Check sheet for the modelled part. Datum: model origin and axes. Units: mm. Face numbers are marked on the shaded views. Give positions to 0.01 mm unless a question says otherwise; leave off trailing zeros. Order: outer loops, then holes, each group sorted by start corner. A loop starts at its lowest first (then second) coordinate and runs counter-clockwise, first axis right, second up.
from build123d import *

# Parameters (mm, degrees)
F3_DEPTH = 1.27


with BuildPart() as f1:
    # F0 (on Front) → F1 (revolve)
    with BuildSketch(Plane.XZ):
        with BuildLine():
            Line((-6.985, 6.35), (-6.985, 0))
            Line((-6.985, 0), (-3.81, 0))
            ThreePointArc((-3.81, 0), (-2.6940768363, 2.6940768363), (0, 3.81))
            Line((0, 3.81), (0, 6.35))
            Line((0, 6.35), (-6.985, 6.35))
        make_face()
    revolve(axis=Axis((0, 0, 5.08), (0, 0, 1)))

    # F2 (on face) → F3 (cut)
    with BuildSketch(Plane.XY.offset(6.35)):
        with BuildLine():
            Line((-5.0499272347, 4.825811841), (5.0499272347, 4.825811841))
            ThreePointArc((5.0499272347, 4.825811841), (0, 6.985), (-5.0499272347, 4.825811841))
        make_face()
        with BuildLine():
            Line((5.0499272347, -4.825811841), (5.0499272347, 4.825811841))
            Line((5.0499272347, 4.825811841), (-5.0499272347, 4.825811841))
            Line((-5.0499272347, 4.825811841), (-5.0499272347, -4.825811841))
            Line((-5.0499272347, -4.825811841), (-1.3193129815, -4.825811841))
            add(Edge.make_bspline(
                [(-1.3193129815, -4.825811841), (-2.5203953314, -4.5677027566), (-3.3083202269, -3.8047253512)],
                knots=[0.3382919108, 0.3382919108, 0.3382919108, 1, 1, 1], degree=2))
            add(Edge.make_bspline(
                [(-3.3083202269, -3.8047253512), (-4.4990641643, -2.6516830689), (-4.4990641643, -0.5382958521)],
                knots=[0, 0, 0, 1, 1, 1], degree=2))
            add(Edge.make_bspline(
                [(-4.4990641643, -0.5382958521), (-4.4990641643, 1.7656941762), (-3.3439273456, 2.9082637766)],
                knots=[0, 0, 0, 1, 1, 1], degree=2))
            add(Edge.make_bspline(
                [(-3.3439273456, 2.9082637766), (-2.1887905268, 4.0508333769), (0.0418907278, 4.0508333769)],
                knots=[0, 0, 0, 1, 1, 1], degree=2))
            add(Edge.make_bspline(
                [(0.0418907278, 4.0508333769), (1.6400219928, 4.0508333769), (3.1250482929, 3.6570605358)],
                knots=[0, 0, 0, 1, 1, 1], degree=2))
            Line((3.1250482929, 3.6570605358), (3.1250482929, 1.7719777854))
            Line((3.1250482929, 1.7719777854), (2.6872901875, 1.7719777854))
            Line((2.6872901875, 1.7719777854), (2.5092545944, 2.8590421714))
            add(Edge.make_bspline(
                [(2.5092545944, 2.8590421714), (2.0589292707, 3.179506239), (1.4274265493, 3.3533527593)],
                knots=[0, 0, 0, 1, 1, 1], degree=2))
            add(Edge.make_bspline(
                [(1.4274265493, 3.3533527593), (0.7959238279, 3.5271992796), (0.0942541375, 3.5271992796)],
                knots=[0, 0, 0, 1, 1, 1], degree=2))
            add(Edge.make_bspline(
                [(0.0942541375, 3.5271992796), (-1.5813749739, 3.5271992796), (-2.356353438, 2.5281054219)],
                knots=[0, 0, 0, 1, 1, 1], degree=2))
            add(Edge.make_bspline(
                [(-2.356353438, 2.5281054219), (-3.131331902, 1.5290115642), (-3.131331902, -0.5257286337)],
                knots=[0, 0, 0, 1, 1, 1], degree=2))
            add(Edge.make_bspline(
                [(-3.131331902, -0.5257286337), (-3.131331902, -2.4568911847), (-2.3333135377, -3.4549377742)],
                knots=[0, 0, 0, 1, 1, 1], degree=2))
            add(Edge.make_bspline(
                [(-2.3333135377, -3.4549377742), (-1.5352951734, -4.4529843637), (0.0293235095, -4.4529843637)],
                knots=[0, 0, 0, 1, 1, 1], degree=2))
            add(Edge.make_bspline(
                [(0.0293235095, -4.4529843637), (0.5801865798, -4.4529843637), (1.1823657918, -4.3220758394)],
                knots=[0, 0, 0, 1, 1, 1], degree=2))
            add(Edge.make_bspline(
                [(1.1823657918, -4.3220758394), (1.7845450037, -4.191167315), (2.0987254621, -4.0068481128)],
                knots=[0, 0, 0, 1, 1, 1], degree=2))
            Line((2.0987254621, -4.0068481128), (2.0987254621, -1.5143498095))
            Line((2.0987254621, -1.5143498095), (0.9718648846, -1.3425978256))
            Line((0.9718648846, -1.3425978256), (0.9718648846, -0.9907157121))
            Line((0.9718648846, -0.9907157121), (4.2121126789, -0.9907157121))
            Line((4.2121126789, -0.9907157121), (4.2121126789, -1.3425978256))
            Line((4.2121126789, -1.3425978256), (3.3554472957, -1.5143498095))
            Line((3.3554472957, -1.5143498095), (3.3554472957, -4.3671083717))
            add(Edge.make_bspline(
                [(3.3554472957, -4.3671083717), (2.5951305864, -4.6163582021), (1.7772141263, -4.7870629178)],
                knots=[0, 0, 0, 1, 1, 1], degree=2))
            add(Edge.make_bspline(
                [(1.7772141263, -4.7870629178), (1.6784160951, -4.8076827374), (1.5777996884, -4.825811841)],
                knots=[0, 0, 0, 0.1207923255, 0.1207923255, 0.1207923255], degree=2))
            Line((1.5777996884, -4.825811841), (5.0499272347, -4.825811841))
        make_face()
        with BuildLine():
            Line((-5.0499272347, -4.825811841), (-5.0499272347, 4.825811841))
            ThreePointArc((-5.0499272347, 4.825811841), (-6.985, 0), (-5.0499272347, -4.825811841))
        make_face()
        with BuildLine():
            ThreePointArc((-5.0499272347, -4.825811841), (0, -6.985), (5.0499272347, -4.825811841))
            Line((5.0499272347, -4.825811841), (1.5777996884, -4.825811841))
            add(Edge.make_bspline(
                [(1.5777996884, -4.825811841), (0.8454459018, -4.9577676335), (0.0167562911, -4.9577676335)],
                knots=[0.1207923255, 0.1207923255, 0.1207923255, 1, 1, 1], degree=2))
            add(Edge.make_bspline(
                [(0.0167562911, -4.9577676335), (-0.7052711558, -4.9577676335), (-1.3193129815, -4.825811841)],
                knots=[0, 0, 0, 0.3382919108, 0.3382919108, 0.3382919108], degree=2))
            Line((-1.3193129815, -4.825811841), (-5.0499272347, -4.825811841))
        make_face()
        with BuildLine():
            ThreePointArc((6.985, 0), (6.4832077992, 2.5996618305), (5.0499272347, 4.825811841))
            Line((5.0499272347, 4.825811841), (5.0499272347, -4.825811841))
            ThreePointArc((5.0499272347, -4.825811841), (6.4832077992, -2.5996618305), (6.985, 0))
        make_face()
    extrude(amount=-F3_DEPTH, mode=Mode.SUBTRACT)


solid = f1.part
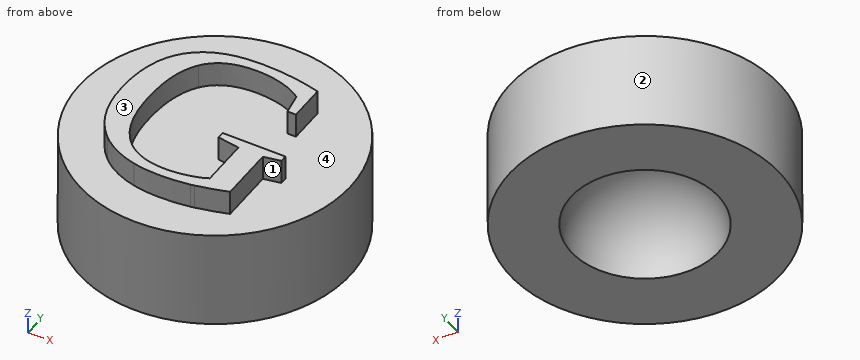
1) Section check B-B, the plane x = -5.5. Record the cut outline in (y, z).
Recorded:
outline: (-4.31, 0) - (4.31, 0) - (4.31, 5.08) - (-4.31, 5.08) - close
2) Draft check along X on the marked faces 1, 2, 3 and 4. Enter one of: +X half, -X half, draft (parallel to the pull), parting line (faces both ways), or undercut.
Recorded:
face 1: +X half
face 2: parting line
face 3: draft
face 4: undercut
3) Section check A-A, the plane z = 3. Record the cut outline in (x, y) (3 decimals).
Recorded:
outline: circle Ø13.97 at (0, 0); hole circle Ø4.697 at (0, 0)
4) Depth check by flat-ended pin: pin 1 Ø1.4 at (x, z) = (3, 5.5) entering from +Y; pin 2 Ø1 at (y, z) = (-2.5, 5.5) entering from +X; pin 3 Ø3 at (x, z) = (2.5, 2.5) entering from +Y. Enter the tip coordinate at first touch or a pass-through.
Recorded:
pin 1: stops at y = 6.54
pin 2: stops at x = 6.62
pin 3: stops at y = 6.91
5) Section check D-D, the plane z = 2.25. Record the cut outline in (x, y) (3 decimals).
Recorded:
outline: circle Ø13.97 at (0, 0); hole circle Ø6.149 at (0, 0)
6) Material ranges on L1, parallel to Y at x = 0.25, z = 1.25; L2, parallel to Z at x = -4.75, y = -1.25; L3, parallel to Y at x = -2.25, z = 0.5, recorded low to high.
Recorded:
L1: y = -6.98 to -3.59, 3.59 to 6.98
L2: z = 0 to 5.08
L3: y = -6.61 to -3.03, 3.03 to 6.61
